Input: part model. Units: mm. Frame: model coordinates. A direction names the side the tool comes from. Give positions to 0.01 mm unless a question says otherwise; leave off trailing zeros. Loops run counter-clockwise (first coordinate to the right, second up) from the corner with the lowest first, then second, coordinate; pieces in that order, holes last. Notation, with made-up numbers: (7.25, -23.5) - (55.25, -23.5) arc R17 ccw to (55.25, -1.5) - close; hole circle Ø11 at (-17.5, 30.25). An arc over 180 degrees is marked (long way). Answer as a JSON object with one key per item and string values. Group by question number.
(1) Section query B-B (y = 12.7). Return loops of the section in (x, z) (3 decimals).
(2) Section query D-D (z = -9.75). Return loops of the section in (x, y) (3 decimals), plus the area to 3 significant figures.
(3) Mould query, pull axis X, two halves, no side actions, for faces 1 (the flat face through (5.2, 9.7, -19.05)), 2 (the cylindrical face through (-13.76, 23.21, -1.61)), 3 (the cylindrical face through (11.157, 12.878, -3.557)). Classes: +X half, -X half, draft (parallel to the pull), parting line (faces both ways), or undercut.
(4) Access query for faces 4 (the flat face through (10.795, 13, -10)), 5 (the flat face through (-10.795, 13, -10)), 6 (the cylindrical face through (-14.847, 5.186, -1.61)). Directions: +Z, -Z, +X, -X, +Y, -Y. A direction counts if a zero-diameter tool reaches every point of the face in a straight line with its end or side. Return the directions, or none.
(5) Pin query (flat end, axial travel): P1, Ø3.5, axis at y = 15, z = -8, coming from the -X side (3 decimals); P2, Ø1.5, axis at x = 13.5, y = 17, coming from the -Z side (3 decimals); P3, Ø5, axis at x = -13.97, y = 3.81, coming from the -Z side; P4, Ø7, axis at x = 0, y = 12.7, coming from the -Z side. Return the tip coordinate at first contact, or that it passes through.
(6) Section query C-C (x = -13.97). Return loops of the section in (y, z) (3 decimals), plus the area to 3 significant figures.
(7) Material intervals for L1, parallel to Y at x = -13.97, z = -1.4; L2, parallel to Z at x = 13.5, y = 6.25 (3 decimals); L3, parallel to X at y = 18.5, z = -9 (3 decimals), sorted ascending.
(8) Section query A-A (x = 0). Return loops of the section in (y, z) (3 decimals).
```python
from build123d import *

# Parameters (mm, degrees)
BOSS_EXTRUDE4_DEPTH = 25.4
CHAMFER1_SIZE       = 3.175
SKETCH10_R          = 1.63195
CUT_EXTRUDE3_DEPTH  = 3.175
SKETCH11_R          = 5.715
CUT_EXTRUDE4_DEPTH  = 20.05
FILLET1_R           = 1.27


with BuildPart() as part:
    # Sketch4 → Boss-Extrude4 (new body)
    with BuildSketch(Plane(origin=(0, 0, 0), x_dir=(1, 0, 0), z_dir=(0, 1, 0))):
        Polygon((-10.795, 3.175), (-17.145, 3.175), (-17.145, 0), (-12.7, 0), (12.7, 0), (17.145, 0), (17.145, 3.175), (10.795, 3.175), (10.795, 19.05), (-10.795, 19.05), align=None)
    extrude(amount=BOSS_EXTRUDE4_DEPTH)

    # Chamfer1
    chamfer1_edges = [part.edges().sort_by_distance(p)[0] for p in [
        (-10.795, 12.7, -19.05),
        (10.795, 12.7, -19.05),
    ]]
    chamfer(chamfer1_edges, length=CHAMFER1_SIZE)

    # Sketch10 → Cut-Extrude3 (cut)
    with BuildSketch(Plane(origin=(0, 0, -3.175), x_dir=(-1, 0, 0), z_dir=(0, 0, -1))):
        with Locations((-13.97, 21.59)):
            Circle(SKETCH10_R)
        with Locations((-13.97, 3.81)):
            Circle(SKETCH10_R)
        with Locations((13.97, 3.81)):
            Circle(SKETCH10_R)
        with Locations((13.97, 21.59)):
            Circle(SKETCH10_R)
    extrude(amount=-CUT_EXTRUDE3_DEPTH, mode=Mode.SUBTRACT)

    # Sketch11 → Cut-Extrude4 (cut, through all)
    with BuildSketch(Plane(origin=(0, 0, -19.05), x_dir=(-1, 0, 0), z_dir=(0, 0, -1))):
        with Locations((0, 12.7)):
            Circle(SKETCH11_R)
    extrude(amount=-CUT_EXTRUDE4_DEPTH, mode=Mode.SUBTRACT)

    # Fillet1
    fillet1_edges = [part.edges().sort_by_distance(p)[0] for p in [
        (-10.795, 12.7, -3.175),
        (10.795, 12.7, -3.175),
    ]]
    fillet(fillet1_edges, radius=FILLET1_R)


solid = part.part
```
Recorded:
{
 "1": {"outline": "(-17.145, -3.175) - (-12.065, -3.175) arc R1.27 cw to (-10.795, -4.445) - (-10.795, -15.875) - (-7.62, -19.05) - (-5.715, -19.05) - (-5.715, 0) - (-17.145, 0) - close; (5.715, -19.05) - (7.62, -19.05) - (10.795, -15.875) - (10.795, -4.445) arc R1.27 cw to (12.065, -3.175) - (17.145, -3.175) - (17.145, 0) - (5.715, 0) - close"},
 "2": {"outline": "(-10.795, 0) - (10.795, 0) - (10.795, 25.4) - (-10.795, 25.4) - close; hole circle Ø11.43 at (0, 12.7)", "area": "446 mm^2"},
 "3": {"face 1": "draft", "face 2": "undercut", "face 3": "+X half"},
 "4": {"face 4": "-Z, +X, +Y, -Y", "face 5": "-Z, -X, +Y, -Y", "face 6": "+Z, -Z"},
 "5": {"P1": "stops at x = -10.795", "P2": "stops at z = -3.175", "P3": "stops at z = -3.32", "P4": "passes through"},
 "6": {"outline": "(0, -3.175) - (2.178, -3.175) - (2.178, 0) - (0, 0) - close; (5.442, -3.175) - (19.958, -3.175) - (19.958, 0) - (5.442, 0) - close; (23.222, -3.175) - (25.4, -3.175) - (25.4, 0) - (23.222, 0) - close", "area": "59.9 mm^2"},
 "7": {"L1": "y = 0 to 2.18, 5.44 to 19.96, 23.22 to 25.4", "L2": "z = -3.175 to 0", "L3": "x = -10.795 to 10.795"},
 "8": {"outline": "(0, -19.05) - (6.985, -19.05) - (6.985, 0) - (0, 0) - close; (18.415, -19.05) - (25.4, -19.05) - (25.4, 0) - (18.415, 0) - close"}
}
